The listing builds one solid part. Answer for the finished solid, in the listing's coordinates (mm). A direction names the side the tool comes from. Round coordinates to 2 decimals unless told otherwise and drop trailing zeros. Order: outer loops, then holes, each group sorted by start corner. A loop starts at its lowest first (then second) coordinate and runs counter-clockwise, first axis right, second up. Notation, with made-up numbers: M -24,6 L -2,6 A25 cw -2,19 Z; hole C 71,-4 d2. An arc over 180 degrees is marked long. Put each result on its own line as item: value. Start each with the question number.
1. The mould has two halves that part along Z. Classify faces 1 (the face through (57.042, -11.619, -28.986)), 2 (the face through (37, 41, -28)): +Z half, -Z half, draft (parallel to the pull), parting line (faces both ways), or undercut.
2. The part is cut by section D-D (x = 101.5). Give the vertices of the cut face in (y, z), then the cut area to 3 significant figures.
3. Each of these flat-tipped pins is pushed along its axis until it touches: pin 1 Ø1.6 at (y, z) = (-4, 50.5) entering from -X; pin 2 Ø12 at (x, z) = (-38.5, 1.5) entering from +Y; pin 3 Ø12 at (x, y) = (-57.5, 8) entering from +Z; pin 4 Ø2 at (y, z) = (22, 38.5) entering from +X. Where does it stop, or does it pass through?
4. The part is cut by section A-A (x = 8). Give the vertices of the cut face in (y, z), then the cut area to 3 significant figures.
5. Consider line 1 (Z direction, x = -28, y = 4); line 2 (X direction, y = 92, z = -8.5); line 3 (Y direction, x = 99.5, z = 45). Determine where each line is inside the solid, lowest interval first.
6. Which of the six approach directions +Z, -Z, +X, -X, +Y, -Y give full straight-line access (tool end or side, diameter ignored) to faces 3 (the face through (95, 18, 0)), 4 (the face through (57.042, -11.619, 29.014)), 5 (the face through (37, 41, 28)), 6 (the face through (0, 87, 0))?
7. The part is cut by section B-B (z = -5.5). Give the vertices of the cut face in (x, y), then the cut area to 3 significant figures.
8. The part is cut by section C-C (y = 43). Give the vertices of the cut face in (x, z), then the cut area to 3 significant figures.
from build123d import *

# Parameters (mm, degrees)
BOSS_EXTRUDE3_DEPTH = 30
SHELL1_T            = -2
BOSS_EXTRUDE2_DEPTH = 25
CUT_EXTRUDE1_REACH  = 172.593
SKETCH5_W           = 35
SKETCH5_H           = 16.5
CUT_EXTRUDE2_REACH  = 173.535
SKETCH6_R           = 1.486127865


with BuildPart() as part:
    # Sketch8 → Boss-Extrude3 (new, symmetric)
    with BuildSketch(Plane.XY):
        Polygon((77, 0), (113, 36), (113, 100), (-2, 100), (-2, 75), (-77, 0), (-77, -20), (60, -20), (54, -3), (54, 0), align=None)
    extrude(amount=BOSS_EXTRUDE3_DEPTH, both=True)

    # Shell1
    shell1_openings = [part.faces().sort_by_distance(p)[0] for p in [
        (54, -1.5, 0),
        (57, -11.5, 0),
        (-8.5, -20, 0),
        (-77, -10, 0),
        (55.5, 100, 0),
        (65.5, 0, 0),
    ]]
    offset(amount=SHELL1_T, openings=shell1_openings, kind=Kind.INTERSECTION)

    # Sketch4 → Boss-Extrude2 (add, symmetric)
    with BuildSketch(Plane(origin=(87, 0, 0), x_dir=(0, 0, -1), z_dir=(1, 0, 0))):
        Polygon((-30, 20), (-30, 18), (-49.58, 18), (-49.58, -10), (-51.58, -10), (-51.58, 20), align=None)
    extrude(amount=BOSS_EXTRUDE2_DEPTH, both=True)

    # Sketch5 → Cut-Extrude1 (cut, up to next)
    with BuildSketch(Plane(origin=(0, 0, 49.58), x_dir=(-1, 0, 0), z_dir=(0, 0, -1)), mode=Mode.PRIVATE) as cut_extrude1_sk1:
        with Locations((-86.503731014, 0)):
            Rectangle(SKETCH5_W, SKETCH5_H)
    cut_extrude1_tool1 = extrude(cut_extrude1_sk1.sketch, amount=-CUT_EXTRUDE1_REACH, mode=Mode.PRIVATE) & part.part
    add(cut_extrude1_tool1.solids().sort_by_distance((86.503731, 0, 49.58))[0], mode=Mode.SUBTRACT)

    # Sketch6 → Cut-Extrude2 (cut, up to next)
    with BuildSketch(Plane.XY.offset(51.58), mode=Mode.PRIVATE) as cut_extrude2_sk1:
        with Locations((66.968636912, 4.723763571)):
            Circle(SKETCH6_R)
    cut_extrude2_tool1 = extrude(cut_extrude2_sk1.sketch, amount=-CUT_EXTRUDE2_REACH, mode=Mode.PRIVATE) & part.part
    # Sketch6 → Cut-Extrude2 (cut, up to next)
    with BuildSketch(Plane.XY.offset(51.58), mode=Mode.PRIVATE) as cut_extrude2_sk2:
        with Locations((106.722557298, 4.723763571)):
            Circle(SKETCH6_R)
    cut_extrude2_tool2 = extrude(cut_extrude2_sk2.sketch, amount=-CUT_EXTRUDE2_REACH, mode=Mode.PRIVATE) & part.part
    # Sketch6 → Cut-Extrude2 (cut, up to next)
    with BuildSketch(Plane.XY.offset(51.58), mode=Mode.PRIVATE) as cut_extrude2_sk3:
        with Locations((106.722557298, -4.723763571)):
            Circle(SKETCH6_R)
    cut_extrude2_tool3 = extrude(cut_extrude2_sk3.sketch, amount=-CUT_EXTRUDE2_REACH, mode=Mode.PRIVATE) & part.part
    # Sketch6 → Cut-Extrude2 (cut, up to next)
    with BuildSketch(Plane.XY.offset(51.58), mode=Mode.PRIVATE) as cut_extrude2_sk4:
        with Locations((66.968636912, -4.723763571)):
            Circle(SKETCH6_R)
    cut_extrude2_tool4 = extrude(cut_extrude2_sk4.sketch, amount=-CUT_EXTRUDE2_REACH, mode=Mode.PRIVATE) & part.part
    add(cut_extrude2_tool1.solids().sort_by_distance((66.968637, 4.723764, 51.58))[0], mode=Mode.SUBTRACT)
    add(cut_extrude2_tool2.solids().sort_by_distance((106.722557, 4.723764, 51.58))[0], mode=Mode.SUBTRACT)
    add(cut_extrude2_tool3.solids().sort_by_distance((106.722557, -4.723764, 51.58))[0], mode=Mode.SUBTRACT)
    add(cut_extrude2_tool4.solids().sort_by_distance((66.968637, -4.723764, 51.58))[0], mode=Mode.SUBTRACT)


solid = part.part
Resolved:
1. face 1: draft
1. face 2: undercut
2. outline: M -10,49.58 L -8.25,49.58 L -8.25,51.58 L -10,51.58 Z; M 8.25,49.58 L 18,49.58 L 18,30 L 20,30 L 20,51.58 L 8.25,51.58 Z; M 24.5,-30 L 100,-30 L 100,-28 L 27.33,-28 L 27.33,28 L 100,28 L 100,30 L 24.5,30 Z
2. area: 527 mm2
3. pin 1: x = 62
3. pin 2: y = 44.5
3. pin 3: z = 30
3. pin 4: through
4. outline: M -20,-30 L 100,-30 L 100,-28 L -20,-28 Z; M -20,28 L 100,28 L 100,30 L -20,30 Z
4. area: 480 mm2
5. line 1: -30 to -28, 28 to 30
5. line 2: -2 to 0, 111 to 113
5. line 3: 18 to 20
6. face 3: -Z, +X, -Y
6. face 4: +Z, -Z, +X
6. face 5: none
6. face 6: +Y, -Y
7. outline: M -77,-2.83 L 0,74.17 L 0,100 L -2,100 L -2,75 L -77,0 Z; M 74.17,0 L 77,0 L 113,36 L 113,100 L 111,100 L 111,36.83 Z
7. area: 496 mm2
8. outline: M -34,-30 L 113,-30 L 113,30 L -34,30 Z; hole M -31.17,-28 L 111,-28 L 111,28 L -31.17,28 Z
8. area: 858 mm2
